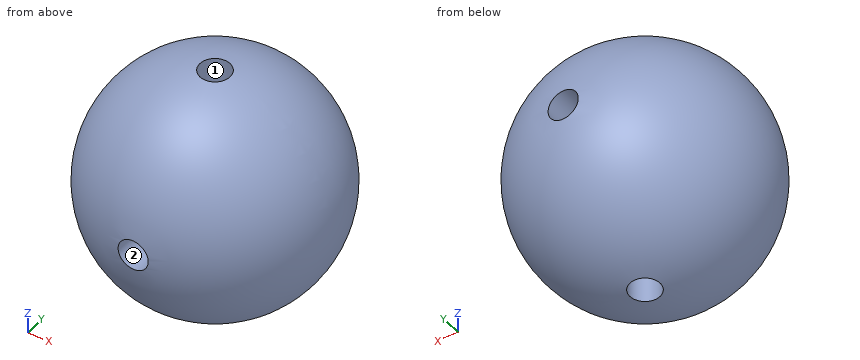
```python
from build123d import *

# Parameters (mm, degrees)
CUT_EXTRUDE3_REACH                  = 15.597
CUT_EXTRUDE3_END_RADIUS             = 7.85
SKETCH3_R                           = 1
CUT_EXTRUDE3_DIRECTION_2_REACH      = 15.597
CUT_EXTRUDE3_DIRECTION_2_END_RADIUS = 7.85
CUT_EXTRUDE4_REACH                  = 15.597
CUT_EXTRUDE4_END_RADIUS             = 7.85
SKETCH4_R                           = 1
CUT_EXTRUDE4_DIRECTION_2_REACH      = 15.597
CUT_EXTRUDE4_DIRECTION_2_END_RADIUS = 7.85


with BuildPart() as part:
    # Sketch2 → Revolve1 (revolve)
    with BuildSketch(Plane(origin=(0, 0, 0), x_dir=(1, 0, 0), z_dir=(0, 1, 0))):
        with BuildLine():
            Line((0, 7.85), (0, -7.85))
            ThreePointArc((0, -7.85), (7.85, 0), (0, 7.85))
        make_face()
    revolve(axis=Axis((0, 0, -7.85), (0, 0, 1)))

    # Cut-Extrude3: up to this sphere (the profile starts inside it)
    cut_extrude3_end = Location((0, 0, 0)) * Sphere(CUT_EXTRUDE3_END_RADIUS, mode=Mode.PRIVATE)
    # Sketch3 → Cut-Extrude3 (cut, up to the surface)
    with BuildSketch(Plane(origin=(0, 0, 0), x_dir=(1, 0, 0), z_dir=(0, 1, 0)), mode=Mode.PRIVATE) as cut_extrude3_sk1:
        with Locations(Location((0, 0, 0), (0, 0, 90))):
            Circle(SKETCH3_R)
    cut_extrude3_tool1 = extrude(cut_extrude3_sk1.sketch, amount=-CUT_EXTRUDE3_REACH, mode=Mode.PRIVATE) & cut_extrude3_end
    add(cut_extrude3_tool1.solids().sort_by_distance((0, 0, 0))[0], mode=Mode.SUBTRACT)

    # Cut-Extrude3 direction 2: up to this sphere (the profile starts inside it)
    cut_extrude3_direction_2_end = Location((0, 0, 0)) * Sphere(CUT_EXTRUDE3_DIRECTION_2_END_RADIUS, mode=Mode.PRIVATE)
    # Sketch3 → Cut-Extrude3 direction 2 (cut, up to the surface)
    with BuildSketch(Plane(origin=(0, 0, 0), x_dir=(1, 0, 0), z_dir=(0, 1, 0)), mode=Mode.PRIVATE) as cut_extrude3_direction_2_sk1:
        with Locations(Location((0, 0, 0), (0, 0, 90))):
            Circle(SKETCH3_R)
    cut_extrude3_direction_2_tool1 = extrude(cut_extrude3_direction_2_sk1.sketch, amount=CUT_EXTRUDE3_DIRECTION_2_REACH, mode=Mode.PRIVATE) & cut_extrude3_direction_2_end
    add(cut_extrude3_direction_2_tool1.solids().sort_by_distance((0, 0, 0))[0], mode=Mode.SUBTRACT)

    # Cut-Extrude4: up to this sphere (the profile starts inside it)
    cut_extrude4_end = Location((0, 0, 0)) * Sphere(CUT_EXTRUDE4_END_RADIUS, mode=Mode.PRIVATE)
    # Sketch4 → Cut-Extrude4 (cut, up to the surface)
    with BuildSketch(Plane.XY, mode=Mode.PRIVATE) as cut_extrude4_sk1:
        Circle(SKETCH4_R)
    cut_extrude4_tool1 = extrude(cut_extrude4_sk1.sketch, amount=-CUT_EXTRUDE4_REACH, mode=Mode.PRIVATE) & cut_extrude4_end
    add(cut_extrude4_tool1.solids().sort_by_distance((0, 0, 0))[0], mode=Mode.SUBTRACT)

    # Cut-Extrude4 direction 2: up to this sphere (the profile starts inside it)
    cut_extrude4_direction_2_end = Location((0, 0, 0)) * Sphere(CUT_EXTRUDE4_DIRECTION_2_END_RADIUS, mode=Mode.PRIVATE)
    # Sketch4 → Cut-Extrude4 direction 2 (cut, up to the surface)
    with BuildSketch(Plane.XY, mode=Mode.PRIVATE) as cut_extrude4_direction_2_sk1:
        Circle(SKETCH4_R)
    cut_extrude4_direction_2_tool1 = extrude(cut_extrude4_direction_2_sk1.sketch, amount=CUT_EXTRUDE4_DIRECTION_2_REACH, mode=Mode.PRIVATE) & cut_extrude4_direction_2_end
    add(cut_extrude4_direction_2_tool1.solids().sort_by_distance((0, 0, 0))[0], mode=Mode.SUBTRACT)


solid = part.part
```
Can you work these out from the model? Positions are in its coordinate system, mm. Face numbers are marked on the shaded views. Coordinates: 2 decimals unless noted, no trailing zeros. Order: outer loops, then holes, each group sorted by start corner. A loop starts at its lowest first (then second) coordinate and runs counter-clockwise, first axis right, second up.
1. Thinking about a two-plate mould opening in Y: for the marked faces 1 and 2, which applies, +Y half, -Y half, draft (parallel to the pull), parting line (faces both ways), or undercut?
2. If we section it at C-C (z = -3.5): Please give me the cut outline in (x, y).
3. If we section it at A-A (x = 0): Please give me the cut outline in (y, z).
4. I'm going to push flat-ended pins straight in: pin 1 (1 mm diameter, centred on x = 6, y = 6, fed in from +Z); pin 2 (4 mm diameter, centred on x = -1.5, y = -4.5, fed in from +Z) (3 decimals); pin 3 (1 mm diameter, centred on x = -1, z = -5, fed in from -Y); pin 4 (1 mm diameter, centred on x = 1, z = 2.5, fed in from -Y). Where does each tip first touch, or does it pass through?
5. If we section it at D-D (y = 1.5): Please give me the cut outline in (x, z), then the cut area to 3 significant figures.
6. If we section it at B-B (x = 4.25): Please give me the cut outline in (y, z).
7. I need wall thicknesses on line 1 (Y direction, x = 0.75, z = 5.5); line 2 (X direction, y = 2.75, z = -0.5); line 3 (Y direction, x = 0, z = 4.25). Which ranges of each line are inside material? Lowest first, please.
Entries:
1. face 1: undercut
1. face 2: draft
2. outline: circle Ø14.05 at (0, 0); hole circle Ø2 at (0, 0)
3. outline: (-7.79, -1) arc R7.85 ccw to (-1, -7.79) - (-1, -1) - close; (-7.79, 1) - (-1, 1) - (-1, 7.79) arc R7.85 ccw to start; (1, -7.79) arc R7.85 ccw to (7.79, -1) - (1, -1) - close; (1, 1) - (7.79, 1) arc R7.85 ccw to (1, 7.79) - close
4. pin 1: passes through
4. pin 2: stops at z = 7.355
4. pin 3: stops at y = -6.36
4. pin 4: stops at y = -7.54
5. outline: circle Ø15.41 at (0, 0); hole circle Ø2 at (0, 0)
5. area: 183 mm2
6. outline: circle Ø13.2 at (0, 0)
7. line 1: y = -5.55 to -0.66, 0.66 to 5.55
7. line 2: x = -7.34 to -0.87, 0.87 to 7.34
7. line 3: y = -6.6 to -1, 1 to 6.6
